from build123d import *

# Parameters (mm, degrees)
SKETCH_1_R          = 9.5
SKETCH_1_R_2        = 2.5
EXTRUDE_1_DEPTH     = 25
SKETCH_2_R          = 4
CUT_EXTRUDE_1_DEPTH = 12.5
FILLET_1_R          = 0.3


with BuildPart() as part:
    # 草图1 → 凸台-拉伸1 (new body)
    with BuildSketch(Plane.XY):
        Circle(SKETCH_1_R)
        Circle(SKETCH_1_R_2, mode=Mode.SUBTRACT)
    extrude(amount=EXTRUDE_1_DEPTH)

    # 草图2 → 切除-拉伸1 (cut)
    with BuildSketch(Plane.XY.offset(25)):
        Circle(SKETCH_2_R)
    extrude(amount=-CUT_EXTRUDE_1_DEPTH, mode=Mode.SUBTRACT)

    # 圆角1
    fillet_1_edges = [part.edges().sort_by_distance(p)[0] for p in [
        (-9.5, 0, 0),
        (-9.5, 0, 25),
    ]]
    fillet(fillet_1_edges, radius=FILLET_1_R)


solid = part.part
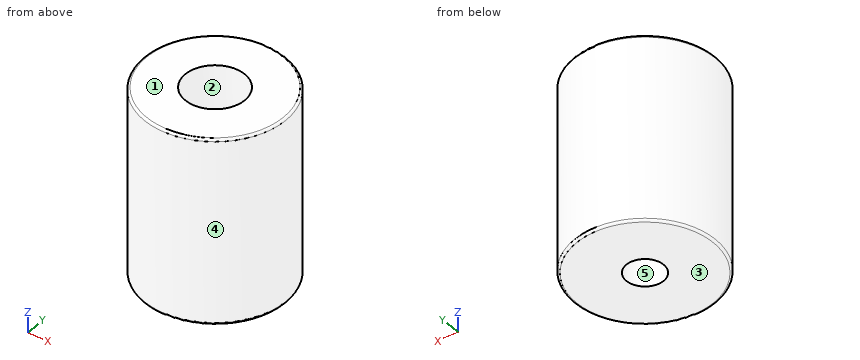
Design review of the part built by this model. Coordinates are the model's own, in mm. Face numbers are marked on the shaded views. A direction names the side the tool comes from. Round coordinates to 2 decimals unless told otherwise and drop trailing zeros. Loops run counter-clockwise (first coordinate to the right, second up) from the corner with the lowest first, then second, coordinate; pieces in that order, holes last. Notation, with made-up numbers: (62, 54.25) - (100, 54.25) arc R17 ccw to (100, 61.25) - close; hole circle Ø8 at (-8.5, 10.25). An arc over 180 degrees is marked (long way). One line per item, written item: value. Start each with the question number.
1) Consider section D-D on z = 15. Give the boundary of the cut face in (x, y).
2) To check wall thickness, follow L1, parallel to Y at x = 0, z = 20.5; L2, parallel to Y at x = 0, z = 7.5; L3, parallel to Z at x = 2.5, y = 1.5. State the ranges of each line that lie inside material, in increasing order. Write a range as from..to.
3) Consider section C-C on z = 10. Give the boundary of the cut face in (x, y).
4) Draft analysis for pull direction X (two halves, no side actions). For the marked faces 3, 4 and 5, state which applies: +X half, -X half, draft (parallel to the pull), parting line (faces both ways), or undercut.
5) Consider section A-A on y = 0. Give the boundary of the cut face in (x, z), then the cut area to 3 significant figures.
6) Insertion check: pin 1 Ø6 at (x, z) = (4, 9) entering from +Y; pin 2 Ø3 at (y, z) = (-3.5, 14) entering from +X; pin 3 Ø3 at (x, z) = (6, 12) entering from -Y. Each pin has a flat end and moves straight along its axis. Give the tip position at first contact, or say it passes through.
7) For the marked faces 1 and 2, list the 3-axis set-ups (+Z, -Z, +X, -X, +Y, -Y) from which the entire face can be reached by the end or side of a thin tool; tool diameter is ignored.
Reported:
1. outline: circle Ø19 at (0, 0); hole circle Ø8 at (0, 0)
2. L1: y = -9.5..-4, 4..9.5
2. L2: y = -9.5..-2.5, 2.5..9.5
2. L3: z = 0..12.5
3. outline: circle Ø19 at (0, 0); hole circle Ø5 at (0, 0)
4. face 3: draft
4. face 4: parting line
4. face 5: undercut
5. outline: (-9.5, 0.3) arc R0.3 ccw to (-9.2, 0) - (-2.5, 0) - (-2.5, 12.5) - (-4, 12.5) - (-4, 25) - (-9.2, 25) arc R0.3 ccw to (-9.5, 24.7) - close; (2.5, 0) - (9.2, 0) arc R0.3 ccw to (9.5, 0.3) - (9.5, 24.7) arc R0.3 ccw to (9.2, 25) - (4, 25) - (4, 12.5) - (2.5, 12.5) - close
5. area: 312 mm^2
6. pin 1: stops at y = 9.45
6. pin 2: stops at x = 9.29
6. pin 3: stops at y = -8.37
7. face 1: +Z, +X, -X, +Y, -Y
7. face 2: +Z
